```python
from build123d import *

# Parameters (mm, degrees)
F0_W     = 95.25
F0_H     = 76.2
F1_DEPTH = 608.0125
F2_W     = 95.25
F2_H     = 95.25
F3_DEPTH = 38.1


with BuildPart() as f1:
    # F0 (on Front) → F1 (new body)
    with BuildSketch(Plane.XZ):
        with Locations((47.625, -38.1)):
            Rectangle(F0_W, F0_H)
    extrude(amount=F1_DEPTH)

    # F2 (on face) → F3 (cut)
    with BuildSketch(Plane.XY):
        with Locations((47.625, -47.625)):
            Rectangle(F2_W, F2_H)
        with Locations((47.625, -382.5875)):
            Rectangle(F2_W, F2_H)
    extrude(amount=-F3_DEPTH, mode=Mode.SUBTRACT)


solid = f1.part
```
The model under review builds one solid part; all positions refer to its coordinate system, in mm. A direction names the side the tool comes from. Round coordinates to 2 decimals unless told otherwise and drop trailing zeros. Write each loop counter-clockwise with the first axis right and the second up, starting at its lowest first coordinate (ties: lowest second). Pieces come first, ordered by that corner, then holes. Notation, with made-up numbers: (57, 41) - (103, 41) arc R27 cw to (103, 67) - close; hole circle Ø1 at (32, 13). An arc over 180 degrees is marked (long way). One line per question, with ' | ' between items.
Item 1: Add section C-C, the plane y = -352. Give the boundary of the cut face in (x, z), then the cut area to 3 significant figures.
Resolved:
outline: (0, -76.2) - (95.25, -76.2) - (95.25, -38.1) - (0, -38.1) - close | area: 3,630 mm2
Item 2: For P1, Ø19, axis at x = 32, z = -24.5, coming from the +Y side; P2, Ø1, axis at x = 48, y = -354.5, coming from the +Z side, all flat-tipped, find the tip position at first contact; note any pin that passes through.
Resolved:
P1: stops at y = -95.25 | P2: stops at z = -38.1
Item 3: Add section A-A, the plane z = -18. Give the boundary of the cut face in (x, y).
Resolved:
outline: (0, -608.01) - (95.25, -608.01) - (95.25, -430.21) - (0, -430.21) - close; (0, -334.96) - (95.25, -334.96) - (95.25, -95.25) - (0, -95.25) - close
Item 4: For faces 4 (the face through (47, -213, 0)), 5 (the face through (47, -95.25, -19)), 6 (the face through (47, -430.212, -19)), list the 3-axis set-ups (+Z, -Z, +X, -X, +Y, -Y) from which the entire face can be reached by the end or side of a thin tool; tool diameter is ignored.
Resolved:
face 4: +Z, +X, -X, +Y, -Y | face 5: +Z, +X, -X, +Y | face 6: +Z, +X, -X
Item 5: The part is to be moulded in two halves that separate along Y. For faces 1 (the face through (0, -300, -39)), 2 (the face through (47, 0, -57)), 3 (the face through (47, -382, -38.1)), say which applies: pulls with the +Y half, pulls with the -Y half, needs draft (parallel to the pull), parting line crosses it, or undercut.
Resolved:
face 1: needs draft | face 2: pulls with the +Y half | face 3: undercut
Item 6: To check wall thickness, follow probe 1 along Y at (x, z) = (68.5, -14.5); probe 2 along Z at (x, y) = (7, -363). State the ranges of each line that lie inside material, in increasing order.
Resolved:
probe 1: y = -608.01 to -430.21, -334.96 to -95.25 | probe 2: z = -76.2 to -38.1
Item 7: Add section B-B, the plane x = 45. Give the boundary of the cut face in (y, z).
Resolved:
outline: (-608.01, -76.2) - (0, -76.2) - (0, -38.1) - (-95.25, -38.1) - (-95.25, 0) - (-334.96, 0) - (-334.96, -38.1) - (-430.21, -38.1) - (-430.21, 0) - (-608.01, 0) - close
